```python
from build123d import *

# Parameters (mm, degrees)
SKETCH1_W               = 34
SKETCH1_H               = 12
BOSS_EXTRUDE1_DEPTH     = 34.00000007
CUT_EXTRUDE_THIN1_DEPTH = 49.456165807
CUT_EXTRUDE1_DEPTH      = 2
SKETCH5_W               = 8.508301653
SKETCH5_H               = 30.00000007
CUT_EXTRUDE2_DEPTH      = 1
CUT_EXTRUDE3_DEPTH      = 50.315688701
CUT_EXTRUDE4_DEPTH      = 49.456165807
BOSS_EXTRUDE2_START     = 1.4
BOSS_EXTRUDE2_DEPTH     = 1.4


with BuildPart() as part:
    # Sketch1 → Boss-Extrude1 (new body)
    with BuildSketch(Plane(origin=(0, 0, 0), x_dir=(1, 0, 0), z_dir=(0, 1, 0))):
        with Locations((17, 0)):
            Rectangle(SKETCH1_W, SKETCH1_H)
    extrude(amount=BOSS_EXTRUDE1_DEPTH)

    # Sketch2 → Cut-Extrude-Thin1 (cut, through all)
    with BuildSketch(Plane.XZ):
        with BuildLine():
            Line((33, -9.62), (10.827001263, -9.62))
            Line((10.827001263, -9.62), (5.81828527, -11.78593124))
            ThreePointArc((5.81828527, -11.78593124), (-3.282636449, -10.995932133), (-7.62, -2.956146555))
            Line((-7.62, -2.956146555), (-7.62, -2.263164725))
            ThreePointArc((-7.62, -2.263164725), (-6.557151524, 2.260930118), (-3.590977529, 5.838484153))
            Line((-3.590977529, 5.838484153), (3.971775857, 11.561648878))
            ThreePointArc((3.971775857, 11.561648878), (6.869113997, 13.091675675), (10.102753387, 13.62))
            Line((10.102753387, 13.62), (33, 13.62))
            ThreePointArc((33, 13.62), (39.095260454, 11.095260454), (41.62, 5))
            Line((41.62, 5), (41.62, -1))
            ThreePointArc((41.62, -1), (39.095260454, -7.095260454), (33, -9.62))
        make_face()
        with BuildLine():
            Line((33, -2), (9.775667088, -2))
            ThreePointArc((9.775667088, -2), (9.260908141, -2.052707652), (8.767512765, -2.208643129))
            Line((8.767512765, -2.208643129), (2.793822301, -4.791860626))
            ThreePointArc((2.793822301, -4.791860626), (0.901738784, -4.627619648), (0, -2.956146555))
            Line((0, -2.956146555), (0, -2.263164725))
            ThreePointArc((0, -2.263164725), (0.265712119, -1.132141014), (1.007255618, -0.237752506))
            Line((1.007255618, -0.237752506), (8.570009004, 5.485412219))
            ThreePointArc((8.570009004, 5.485412219), (9.294343539, 5.867918919), (10.102753387, 6))
            Line((10.102753387, 6), (33, 6))
            ThreePointArc((33, 6), (33.707106781, 5.707106781), (34, 5))
            Line((34, 5), (34, -1))
            ThreePointArc((34, -1), (33.707106781, -1.707106781), (33, -2))
        make_face(mode=Mode.SUBTRACT)
    extrude(amount=-CUT_EXTRUDE_THIN1_DEPTH, mode=Mode.SUBTRACT)

    # Sketch3 → Cut-Extrude1 (cut)
    with BuildSketch(Plane(origin=(0.481189039, 0, -0.635856944), x_dir=(0.7974063856023161, 0, 0.6034426701855364), z_dir=(-0.6034426701855365, 0, 0.7974063856023162))):
        with BuildLine():
            Line((-2.189052199, 32.00000007), (7.310947801, 32.00000007))
            ThreePointArc((7.310947801, 32.00000007), (8.018054582, 31.707106851), (8.310947801, 31.00000007))
            Line((8.310947801, 31.00000007), (8.310947801, 3))
            ThreePointArc((8.310947801, 3), (8.018054582, 2.292893219), (7.310947801, 2))
            Line((7.310947801, 2), (-2.189052199, 2))
            Line((-2.189052199, 2), (-2.189052199, 32.00000007))
        make_face()
    extrude(amount=-CUT_EXTRUDE1_DEPTH, mode=Mode.SUBTRACT)

    # Sketch5 → Cut-Extrude2 (cut)
    with BuildSketch(Plane(origin=(2.185846154, 0, -5.054769231), x_dir=(-0.9178570359601427, 0, -0.39691115068546684), z_dir=(0.39691115068546684, 0, -0.9178570359601427))):
        with Locations((-2.916537368, 17.000000035)):
            Rectangle(SKETCH5_W, SKETCH5_H)
    extrude(amount=-CUT_EXTRUDE2_DEPTH, mode=Mode.SUBTRACT)

    # Sketch6 → Cut-Extrude3 (cut, through all)
    with BuildSketch(Plane.XY.offset(6)):
        with BuildLine():
            Line((5.108391885, 32.00000007), (6.108391885, 32.00000007))
            ThreePointArc((6.108391885, 32.00000007), (6.815498667, 31.707106851), (7.108391885, 31.00000007))
            Line((7.108391885, 31.00000007), (7.108391885, 3))
            ThreePointArc((7.108391885, 3), (6.815498667, 2.292893219), (6.108391885, 2))
            Line((6.108391885, 2), (5.108391885, 2))
            ThreePointArc((5.108391885, 2), (4.401285104, 2.292893219), (4.108391885, 3))
            Line((4.108391885, 3), (4.108391885, 31.00000007))
            ThreePointArc((4.108391885, 31.00000007), (4.401285104, 31.707106851), (5.108391885, 32.00000007))
        make_face()
        with BuildLine():
            Line((10, 34.00000007), (27, 34.00000007))
            Line((27, 34.00000007), (24.899542929, 28.635409633))
            ThreePointArc((24.899542929, 28.635409633), (24.532028014, 28.173988436), (23.968374946, 28.00000007))
            Line((23.968374946, 28.00000007), (15.468374946, 28.00000007))
            ThreePointArc((15.468374946, 28.00000007), (15.04421955, 28.094410649), (14.700153666, 28.35981567))
            Line((14.700153666, 28.35981567), (10, 34.00000007))
        make_face()
        with BuildLine():
            Line((10, 0), (14.700153666, 5.6401844))
            ThreePointArc((14.700153666, 5.6401844), (15.04421955, 5.905589421), (15.468374946, 6))
            Line((15.468374946, 6), (22.925629668, 6))
            ThreePointArc((22.925629668, 6), (23.423690394, 5.867142153), (23.789408568, 5.503871026))
            Line((23.789408568, 5.503871026), (27, 0))
            Line((27, 0), (10, 0))
        make_face()
    extrude(amount=-CUT_EXTRUDE3_DEPTH, mode=Mode.SUBTRACT)

    # Sketch7 → Cut-Extrude4 (cut, through all)
    with BuildSketch(Plane(origin=(34, 0, 0), x_dir=(0, 0, -1), z_dir=(1, 0, 0))):
        with BuildLine():
            Line((-2.75, 32.50000007), (-1.25, 32.50000007))
            ThreePointArc((-1.25, 32.50000007), (0.164213562, 31.914213632), (0.75, 30.50000007))
            Line((0.75, 30.50000007), (0.75, 3.5))
            ThreePointArc((0.75, 3.5), (0.164213562, 2.085786438), (-1.25, 1.5))
            Line((-1.25, 1.5), (-2.75, 1.5))
            ThreePointArc((-2.75, 1.5), (-4.164213562, 2.085786438), (-4.75, 3.5))
            Line((-4.75, 3.5), (-4.75, 30.50000007))
            ThreePointArc((-4.75, 30.50000007), (-4.164213562, 31.914213632), (-2.75, 32.50000007))
        make_face()
    extrude(amount=-CUT_EXTRUDE4_DEPTH, mode=Mode.SUBTRACT)

    # Sketch8 → Boss-Extrude2 (add)
    with BuildSketch(Plane.XZ.offset(BOSS_EXTRUDE2_START)):
        with BuildLine():
            Line((27, 6), (27, -2))
            Line((27, -2), (33, -2))
            ThreePointArc((33, -2), (33.707106781, -1.707106781), (34, -1))
            Line((34, -1), (34, 5))
            ThreePointArc((34, 5), (33.707106781, 5.707106781), (33, 6))
            Line((33, 6), (27, 6))
        make_face()
        with BuildLine():
            Line((10, -2), (10, 5.997920752))
            ThreePointArc((10, 5.997920752), (9.245793944, 5.851070997), (8.570009004, 5.485412219))
            Line((8.570009004, 5.485412219), (1.007255618, -0.237752506))
            ThreePointArc((1.007255618, -0.237752506), (0.265712119, -1.132141014), (0, -2.263164725))
            Line((0, -2.263164725), (0, -2.956146555))
            ThreePointArc((0, -2.956146555), (0.901738784, -4.627619648), (2.793822301, -4.791860626))
            Line((2.793822301, -4.791860626), (8.767512765, -2.208643129))
            ThreePointArc((8.767512765, -2.208643129), (9.260908141, -2.052707652), (9.775667088, -2))
            Line((9.775667088, -2), (10, -2))
        make_face()
    boss_extrude2 = extrude(amount=-BOSS_EXTRUDE2_DEPTH)

    # Mirror1: Boss-Extrude2 across plane
    add(boss_extrude2.mirror(Plane(origin=(0, 17.000000035, 0), x_dir=(0, 0, 1), z_dir=(0, -1, 0))))


solid = part.part
```
Work out the finished part from the listing and answer in its coordinate system (mm). A direction names the side the tool comes from. Coordinates: 2 decimals unless noted, no trailing zeros. Loops run counter-clockwise (first coordinate to the right, second up) from the corner with the lowest first, then second, coordinate; pieces in that order, holes last. Notation, with made-up numbers: (57.25, -28) - (83.25, -28) arc R9 cw to (83.25, -14) - close; hole circle Ø4 at (71.5, -6). An arc over 180 degrees is marked (long way). Use a Markdown table: item, result.
Item 1: The mould has two halves that part along Z. Classify faces 4 (the cylindrical face through (29.54, 2.07, 4.15)), 5 (the flat face through (7.85, 16.91, 4.94)), 6 (the flat face through (6, 35.4, -1)): +Z half, -Z half, draft (parallel to the pull), parting line (faces both ways), or undercut.
Evaluation:
| item | result |
|---|---|
| face 4 | undercut |
| face 5 | +Z half |
| face 6 | draft |
Item 2: Given pin 1 Ø4 at (y, z) = (24.5, 3) entering from -X; pin 2 Ø6 at (x, y) = (29, 8.5) entering from -Z; pin 3 Ø0.6 at (x, z) = (19, -1) entering from -Y, each flat-ended and moving along its own axis, determine where each tip first touches the part or whether it passes through.
Evaluation:
| item | result |
|---|---|
| pin 1 | stops at x = 7.6 |
| pin 2 | stops at z = -2 |
| pin 3 | stops at y = 6 |
Item 3: Find section C-C, the plane z = 2. Determine the outline of the cut face in (x, y) (3 decimals), and give its area (3 significant figures).
Evaluation:
| item | result |
|---|---|
| outline | (3.964, -1.4) - (10, -1.4) - (10, 0) - (11.25, 1.5) - (3.964, 1.5) - close; (3.964, 32.5) - (11.25, 32.5) - (10, 34) - (10, 35.4) - (3.964, 35.4) - close; (26.125, 1.5) - (27, 0) - (27, -1.4) - (34, -1.4) - (34, 1.5) - close; (26.413, 32.5) - (34, 32.5) - (34, 35.4) - (27, 35.4) - (27, 34) - close |
| area | 78.6 mm2 |
Item 4: Consider probe 1 along Z at (x, y) = (14.5, 24.5); probe 2 along Y at (x, z) = (5, -3.5). Determine where each line is inside the solid, lowest interval first. Write a range as from..to.
Evaluation:
| item | result |
|---|---|
| probe 1 | z = -2..-0.75, 4.75..6 |
| probe 2 | y = -1.4..2, 32..35.4 |
Item 5: For faces 1 (the flat face through (19, 6, -1)), 2 (the cylindrical face through (29.87, 31.9, 4.18)), 3 (the cylindrical face through (24.54, 28.18, 5.38)), determine the directions among +Z, -Z, +X, -X, +Y, -Y from which every point of the face is accessible in a straight line to the end or side of a thin tool.
Evaluation:
| item | result |
|---|---|
| face 1 | +Z, -Z, -Y |
| face 2 | +X, -X |
| face 3 | +Z, -Z, +Y |
Item 6: Find section A-A, the plane y = 20. Determine the outline of the cut face in (x, z).
Evaluation:
| item | result |
|---|---|
| outline | (0.06, -3.46) arc R2 ccw to (0.81, -4.56) - (4.11, -3.13) - (4.11, -0.75) - (3.64, -0.75) - close; (7.11, -1.84) - (8.37, -1.29) - (8.77, -2.21) arc R2.54 cw to (9.78, -2) - (33, -2) arc R1 ccw to (34, -1) - (34, -0.75) - (7.11, -0.75) - close; (7.6, 4.75) - (34, 4.75) - (34, 5) arc R1 ccw to (33, 6) - (10.1, 6) arc R2.54 ccw to (8.57, 5.49) - close |
Item 7: Find section D-D, the plane y = 5. Determine the outline of the cut face in (x, z).
Evaluation:
| item | result |
|---|---|
| outline | (0.06, -3.46) arc R2 ccw to (0.81, -4.56) - (4.11, -3.13) - (4.11, -0.75) - (3.64, -0.75) - close; (7.11, -1.84) - (8.37, -1.29) - (8.77, -2.21) arc R2.54 cw to (9.78, -2) - (14.17, -2) - (14.17, -0.75) - (7.11, -0.75) - close; (7.6, 4.75) - (14.17, 4.75) - (14.17, 6) - (10.1, 6) arc R2.54 ccw to (8.57, 5.49) - close; (24.08, -2) - (33, -2) arc R1 ccw to (34, -1) - (34, -0.75) - (24.08, -0.75) - close; (24.08, 4.75) - (34, 4.75) - (34, 5) arc R1 ccw to (33, 6) - (24.08, 6) - close |
Item 8: Find section B-B, the plane x = 17. Determine the outline of the cut face in (y, z).
Evaluation:
| item | result |
|---|---|
| outline | (6, -2) - (28, -2) - (28, -0.75) - (6, -0.75) - close; (6, 4.75) - (28, 4.75) - (28, 6) - (6, 6) - close |
